Geometry: final body of the model. Coordinates: model frame, mm. A direction names the side the tool comes from. Give positions to 0.01 mm unless a question says otherwise; leave off trailing zeros. Write each loop counter-clockwise with the first axis right and the second up, starting at its lowest first coordinate (ties: lowest second). Pieces come first, ordered by that corner, then holes. Notation, with made-up numbers: (23.5, 10.25) -> (40.5, 10.25) arc R30 cw to (40.5, 39.25) -> close; hole circle Ø4 at (70.5, 7.5). An arc over 180 degrees is marked (long way). Use CSV: the item, a comma, the result in double quotes. Start each with the question number.
1) Contact query for flat-ended pins moving along their axis: P1, Ø5, axis at x = 16.5, y = 44, coming from the +Z side; P2, Ø1, axis at y = 45.5, z = 5.5, coming from the +X side; P3, Ø1.5, axis at x = 37.5, y = 37, coming from the +Z side; P4, Ø6.5, axis at x = 22.5, y = 45, coming from the -Z side. Output: stop coordinate, or through.
2) Section B-B (y = 11.5). Output: boundary loops of the cut face in (x, z).
3) Section A-A (z = 15.5). Output: boundary loops of the cut face in (x, y), plus the area to 3 significant figures.
4) Material intervals for line 1 (Y direction, x = 37, z = 36.4); line 2 (Z direction, x = 4.5, y = 38.5); line 3 (Z direction, x = 18, y = 15.5), sorted ascending. Write a range as [from, to].
5) Section C-C (x = 14). Output: boundary loops of the cut face in (y, z).
6) Draft query along X for faces 1 (the face through (4, 3, 18)), 2 (the face through (30.489, 45, 6)), 3 (the face through (21, 22.413, 55)), 4 (the face through (35.8, 4.1, 36.5)). Return one class per face: pulls with the +X half, pulls with the -X half, needs draft (parallel to the pull), parting line crosses it, or undercut.
7) Set-up query: faces 5 (the face through (21, 23, 0)), 6 (the face through (12.22, 45, 6)), 7 (the face through (3, 39, 27)), 8 (the face through (35.8, 36.1, 36.5)). Return all of +Z, -Z, +X, -X, +Y, -Y with unobstructed straight access to the full face (end or side cutting, diameter ignored); none if empty.
8) Section D-D (y = 21). Output: boundary loops of the cut face in (x, z), plus the area to 3 significant figures.
```python
from build123d import *

# Parameters (mm, degrees)
EXTRUDE_1_DEPTH     = 39
CUT_EXTRUDE_1_DEPTH = 18.5
SKETCH_3_R          = 11
EXTRUDE_2_DEPTH     = 2
SKETCH_4_R          = 2.5
EXTRUDE_3_DEPTH     = 22
CUT_EXTRUDE_2_DEPTH = 16
SKETCH_6_R          = 1.5
CUT_EXTRUDE_3_DEPTH = 5
SKETCH_7_W          = 16
SKETCH_7_H          = 4.2
EXTRUDE_4_DEPTH     = 4
SKETCH_8_W          = 18.978516406
SKETCH_8_H          = 3.428953429
SKETCH_8_W_2        = 17.559561908
SKETCH_8_H_2        = 1.773693122
EXTRUDE_5_DEPTH     = 6
SKETCH_9_W          = 11.707219222
SKETCH_9_H          = 3.341648532
CUT_EXTRUDE_4_DEPTH = 2


with BuildPart() as part:
    # 草图1 → 凸台-拉伸1 (new body)
    with BuildSketch(Plane.XY):
        Polygon((0, 37), (5, 42), (37, 42), (42, 37), (42, 5), (37, 0), (5, 0), (0, 5), align=None)
    extrude(amount=EXTRUDE_1_DEPTH)

    # 草图2 → 切除-拉伸1 (cut)
    with BuildSketch(Plane.XY.offset(27)):
        Polygon((37, 42), (35, 42), (42, 35), (42, 37), align=None)
        Polygon((5, 42), (0, 37), (0, 35), (7, 42), align=None)
        Polygon((5, 0), (7, 0), (0, 7), (0, 5), align=None)
        Polygon((37, 0), (42, 5), (42, 7), (35, 0), align=None)
    extrude(amount=-CUT_EXTRUDE_1_DEPTH, mode=Mode.SUBTRACT)

    # 草图3 → 凸台-拉伸2 (add)
    with BuildSketch(Plane.XY.offset(39)):
        with Locations((21, 21)):
            Circle(SKETCH_3_R)
    extrude(amount=EXTRUDE_2_DEPTH)

    # 草图4 → 凸台-拉伸3 (add)
    with BuildSketch(Plane.XY.offset(41)):
        with Locations((21, 21)):
            Circle(SKETCH_4_R)
    extrude(amount=EXTRUDE_3_DEPTH)

    # 草图5 → 切除-拉伸2 (cut)
    with BuildSketch(Plane.XY.offset(63)):
        with BuildLine():
            Line((18.937577059, 22.412944307), (23.062422941, 22.412944307))
            ThreePointArc((23.062422941, 22.412944307), (21, 23.5), (18.937577059, 22.412944307))
        make_face()
    extrude(amount=-CUT_EXTRUDE_2_DEPTH, mode=Mode.SUBTRACT)

    # 草图6 → 切除-拉伸3 (cut)
    with BuildSketch(Plane.XY.offset(39)):
        with Locations((37, 5)):
            Circle(SKETCH_6_R)
        with Locations((5, 5)):
            Circle(SKETCH_6_R)
        with Locations((37, 37)):
            Circle(SKETCH_6_R)
        with Locations((5, 37)):
            Circle(SKETCH_6_R)
    extrude(amount=-CUT_EXTRUDE_3_DEPTH, mode=Mode.SUBTRACT)

    # 草图7 → 凸台-拉伸4 (add)
    with BuildSketch(Plane(origin=(0, 42, 0), x_dir=(1, 0, 0), z_dir=(0, 1, 0))):
        with Locations((21, -2.1)):
            Rectangle(SKETCH_7_W, SKETCH_7_H)
    extrude(amount=EXTRUDE_4_DEPTH)

    # 草图8 → 凸台-拉伸5 (add)
    with BuildSketch(Plane(origin=(0, 42, 0), x_dir=(1, 0, 0), z_dir=(0, 1, 0))):
        with Locations((21, -5.914476715)):
            Rectangle(SKETCH_8_W, SKETCH_8_H)
        with Locations((21, -5.914476714)):
            Rectangle(SKETCH_8_W_2, SKETCH_8_H_2, mode=Mode.SUBTRACT)
    extrude(amount=EXTRUDE_5_DEPTH)

    # 草图9 → 切除-拉伸4 (cut)
    with BuildSketch(Plane.XY.offset(7.628953429)):
        with Locations((21, 46.329175734)):
            Rectangle(SKETCH_9_W, SKETCH_9_H)
    extrude(amount=-CUT_EXTRUDE_4_DEPTH, mode=Mode.SUBTRACT)


solid = part.part
```
Answers follow:
1,P1,"stops at z = 39"
1,P2,"stops at x = 30.49"
1,P3,"stops at z = 34"
1,P4,"stops at z = 0"
2,outline,"(0, 0) -> (42, 0) -> (42, 39) -> (26.55, 39) -> (26.55, 41) -> (15.45, 41) -> (15.45, 39) -> (0, 39) -> close"
3,outline,"(0, 7) -> (7, 0) -> (35, 0) -> (42, 7) -> (42, 35) -> (35, 42) -> (7, 42) -> (0, 35) -> close"
3,area,"1,670 mm^2"
4,line 1,"y = [0, 3.5], [6.5, 35.5], [38.5, 42]"
4,line 2,"z = [0, 39]"
4,line 3,"z = [0, 41]"
5,outline,"(0, 0) -> (46, 0) -> (46, 4.2) -> (48, 4.2) -> (48, 5.03) -> (42, 5.03) -> (42, 6.8) -> (48, 6.8) -> (48, 7.63) -> (42, 7.63) -> (42, 39) -> (29.49, 39) -> (29.49, 41) -> (12.51, 41) -> (12.51, 39) -> (0, 39) -> close"
6,face 1,"pulls with the -X half"
6,face 2,"pulls with the +X half"
6,face 3,"needs draft"
6,face 4,"undercut"
7,face 5,"-Z, +X, -X, +Y, -Y"
7,face 6,"+Y"
7,face 7,"-X, +Y"
7,face 8,"+Z"
8,outline,"(0, 0) -> (42, 0) -> (42, 39) -> (32, 39) -> (32, 41) -> (23.5, 41) -> (23.5, 63) -> (18.5, 63) -> (18.5, 41) -> (10, 41) -> (10, 39) -> (0, 39) -> close"
8,area,"1,790 mm^2"
